from build123d import *

# Parameters (mm, degrees)
F0_W     = 59.521824
F0_H     = 35.536878
F1_DEPTH = 50.8
F2_W     = 45.72
F2_H     = 54.441824
F3_DEPTH = 33.528
F4_R     = 5.08
F5_R     = 5.08
F6_R     = 5.08
F7_SIZE  = 2.54
F8_SIZE  = 2.54
F9_SIZE  = 2.54


with BuildPart() as f1:
    # F0 (on Right) → F1 (new body)
    with BuildSketch(Plane.YZ):
        with Locations((-0.097901, 17.768439)):
            Rectangle(F0_W, F0_H)
    extrude(amount=F1_DEPTH)

    # F2 (on face) → F3 (cut)
    with BuildSketch(Plane.XY.offset(35.536878)):
        with Locations((25.4, -0.097901)):
            Rectangle(F2_W, F2_H)
    extrude(amount=-F3_DEPTH, mode=Mode.SUBTRACT)

    # F4
    f4_edges = [f1.edges().sort_by_distance(p)[0] for p in [
        (0, 29.663011, 17.768439),
        (0, -29.858813, 17.768439),
    ]]
    fillet(f4_edges, radius=F4_R)

    # F5
    f5_edges = [f1.edges().sort_by_distance(p)[0] for p in [
        (50.8, -29.858813, 17.768439),
    ]]
    fillet(f5_edges, radius=F5_R)

    # F6
    f6_edges = [f1.edges().sort_by_distance(p)[0] for p in [
        (50.8, 29.663011, 17.768439),
    ]]
    fillet(f6_edges, radius=F6_R)

    # F7
    f7_edges = [f1.edges().sort_by_distance(p)[0] for p in [
        (48.26, 27.123011, 18.772878),
        (2.54, 27.123011, 18.772878),
    ]]
    chamfer(f7_edges, length=F7_SIZE)

    # F8
    f8_edges = [f1.edges().sort_by_distance(p)[0] for p in [
        (48.26, -27.318813, 18.772878),
        (2.54, -27.318813, 18.772878),
    ]]
    chamfer(f8_edges, length=F8_SIZE)

    # F9
    f9_edges = [f1.edges().sort_by_distance(p)[0] for p in [
        (50.8, -0.097901, 0),
        (49.312102, 28.175114, 0),
        (49.312102, -28.370915, 0),
        (25.4, 29.663011, 0),
        (25.4, -29.858813, 0),
        (1.487898, 28.175114, 0),
        (1.487898, -28.370915, 0),
        (0, -0.097901, 0),
    ]]
    chamfer(f9_edges, length=F9_SIZE)


solid = f1.part
For this review, take the finished solid that the model builds, in its own axes (mm). A direction names the side the tool comes from. Round coordinates to 2 decimals unless told otherwise and drop trailing zeros. Order: outer loops, then holes, each group sorted by start corner. A loop starts at its lowest first (then second) coordinate and runs counter-clockwise, first axis right, second up. Notation, with made-up numbers: M 48,29.5 L 67,29.5 A21 ccw 67,44.5 Z; hole C 9.5,43.5 d5. An arc over 180 degrees is marked long. Write each question's results on one line, items separated by ' | '. Start each with the question number.
1. Draft analysis for pull direction X (two halves, no side actions). For faces 3 (the face through (25.684, 28.375, 1.252)), 4 (the face through (48.17, -27.29, 0.97)), 5 (the face through (1.449, 28.135, 19.269)), 6 (the face through (3.79, -26.03, 19.01)), state which applies: pulls with the +X half, pulls with the -X half, needs draft (parallel to the pull), parting line crosses it, or undercut.
2. Add section C-C (y = -3.5). State the section outline as (x, z) points, then the cut area to 3 significant figures.
3. Add section B-B (x = 26). State the section outline as (y, z) points.
4. Add section A-A (z = 12.5). State the section outline as (x, y) points.
5. To check wall thickness, follow L1, parallel to Y at x = 23, z = 31.5; L2, parallel to X at y = -1, z = 4; L3, parallel to Z at x = 33.5, y = 26. State the ranges of each line that lie inside material, in increasing order. Write a range as [from, to].
6. Tool access review of faces 1 (the face through (25, 0, 0)), 2 (the face through (25, -27.319, 19)): name each direction out of +Z, -Z, +X, -X, +Y, -Y from which nothing blocks a thin tool from reaching the whole face with its end or side.
7. Clearance check with a flat-ended pin moving along its axis: pin 1 Ø1 at (x, y) = (33, -23) entering from +Z. State where the tip first meets the part, or that it passes through.
Output values:
1) face 3: needs draft | face 4: pulls with the +X half | face 5: pulls with the -X half | face 6: undercut
2) outline: M 0,2.54 L 2.54,0 L 48.26,0 L 50.8,2.54 L 50.8,35.54 L 48.26,35.54 L 48.26,2.01 L 2.54,2.01 L 2.54,35.54 L 0,35.54 Z | area: 266 mm^2
3) outline: M -29.86,2.54 L -27.32,0 L 27.12,0 L 29.66,2.54 L 29.66,35.54 L 27.12,35.54 L 27.12,2.01 L -27.32,2.01 L -27.32,35.54 L -29.86,35.54 Z
4) outline: M 0,-24.78 A5.08 ccw 5.08,-29.86 L 45.72,-29.86 A5.08 ccw 50.8,-24.78 L 50.8,24.58 A5.08 ccw 45.72,29.66 L 5.08,29.66 A5.08 ccw 0,24.58 Z; hole M 2.54,-24.78 L 5.08,-27.32 L 45.72,-27.32 L 48.26,-24.78 L 48.26,24.58 L 45.72,27.12 L 5.08,27.12 L 2.54,24.58 Z
5) L1: [-29.86, -27.32], [27.12, 29.66] | L2: [0, 2.54], [48.26, 50.8] | L3: [0, 2.01]
6) face 1: -Z, +X, -X, +Y, -Y | face 2: +Z
7) pin 1: z = 2.01
